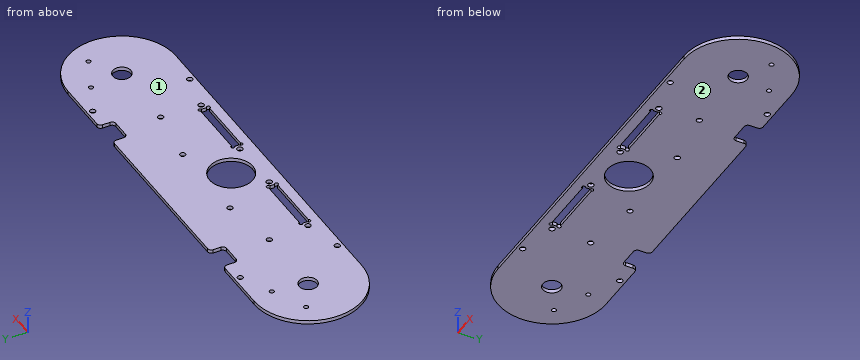
from build123d import *

# Parameters (mm, degrees)
EXTRUDE_1_DEPTH     = 2
SKETCH_2_R          = 1.55
SKETCH_2_R_2        = 12
SKETCH_2_R_3        = 5.025
SKETCH_2_R_4        = 1.25
CUT_EXTRUDE_1_DEPTH = 130.537639318
SKETCH_3_R          = 1.6
SKETCH_3_W          = 34
SKETCH_3_H          = 5
CUT_EXTRUDE_2_DEPTH = 130.537639318
SKETCH_4_W          = 14
SKETCH_4_H          = 8.3
CUT_EXTRUDE_3_DEPTH = 130.537639318
FILLET_1_R          = 2
SKETCH_5_R          = 1
CUT_EXTRUDE_4_DEPTH = 130.537639318


with BuildPart() as part:
    # ｽｹｯﾁ1 → ﾎﾞｽ - 押し出し1 (new body)
    with BuildSketch(Plane.XY):
        with BuildLine():
            Line((-96, -30), (96, -30))
            ThreePointArc((96, -30), (126, 0), (96, 30))
            Line((96, 30), (-96, 30))
            ThreePointArc((-96, 30), (-126, 0), (-96, -30))
        make_face()
    extrude(amount=EXTRUDE_1_DEPTH)

    # ｽｹｯﾁ2 → ｶｯﾄ - 押し出し1 (cut, through all)
    with BuildSketch(Plane.XY.offset(2)):
        with Locations((-56, 0)):
            Circle(SKETCH_2_R)
        with Locations(Location((56, 0, 0), (0, 0, 180))):
            Circle(SKETCH_2_R)
        with Locations((-76, 27)):
            Circle(SKETCH_2_R)
        with Locations((-76, -27)):
            Circle(SKETCH_2_R)
        with Locations(Location((76, 27, 0), (0, 0, 180))):
            Circle(SKETCH_2_R)
        with Locations(Location((76, -27, 0), (0, 0, 180))):
            Circle(SKETCH_2_R)
        with Locations((-24.362267564, 4.80144627)):
            Circle(SKETCH_2_R)
        with Locations(Location((24.362267564, 4.80144627, 0), (0, 0, 180))):
            Circle(SKETCH_2_R)
        with Locations((0, -9)):
            Circle(SKETCH_2_R_2)
        with Locations((-96, 0)):
            Circle(SKETCH_2_R_3)
        with Locations((96, 0)):
            Circle(SKETCH_2_R_3)
        with Locations((-112.152077461, 9.846364808)):
            Circle(SKETCH_2_R_4)
        with Locations((-93.160397784, 18.702330483)):
            Circle(SKETCH_2_R_4)
        with Locations(Location((93.160397784, 18.702330483, 0), (0, 0, 180))):
            Circle(SKETCH_2_R_4)
        with Locations(Location((112.152077461, 9.846364808, 0), (0, 0, 180))):
            Circle(SKETCH_2_R_4)
    extrude(amount=-CUT_EXTRUDE_1_DEPTH, mode=Mode.SUBTRACT)

    # ｽｹｯﾁ3 → ｶｯﾄ - 押し出し2 (cut, through all)
    with BuildSketch(Plane.XY.offset(2)):
        with Locations((55.057299255, -22)):
            Circle(SKETCH_3_R)
        with Locations((15.057299255, -22)):
            Circle(SKETCH_3_R)
        with Locations(Location((-55.057299255, -22, 0), (0, 0, 180))):
            Circle(SKETCH_3_R)
        with Locations(Location((-15.057299255, -22, 0), (0, 0, 180))):
            Circle(SKETCH_3_R)
        with Locations((35.057299255, -22)):
            Rectangle(SKETCH_3_W, SKETCH_3_H)
        with Locations((-35.057299255, -22)):
            Rectangle(SKETCH_3_W, SKETCH_3_H)
    extrude(amount=-CUT_EXTRUDE_2_DEPTH, mode=Mode.SUBTRACT)

    # ｽｹｯﾁ4 → ｶｯﾄ - 押し出し3 (cut, through all)
    with BuildSketch(Plane.XY.offset(2)):
        with Locations((-57.057299255, 25.85)):
            Rectangle(SKETCH_4_W, SKETCH_4_H)
        with Locations((57.057299255, 25.85)):
            Rectangle(SKETCH_4_W, SKETCH_4_H)
    extrude(amount=-CUT_EXTRUDE_3_DEPTH, mode=Mode.SUBTRACT)

    # ﾌｨﾚｯﾄ1
    fillet_1_edges = [part.edges().sort_by_distance(p)[0] for p in [
        (-64.057299255, 21.7, 1),
        (-64.057299255, 30, 1),
        (-50.057299255, 30, 1),
        (-50.057299255, 21.7, 1),
        (50.057299255, 21.7, 1),
        (50.057299255, 30, 1),
        (64.057299255, 30, 1),
        (64.057299255, 21.7, 1),
    ]]
    fillet(fillet_1_edges, radius=FILLET_1_R)

    # ｽｹｯﾁ5 → ｶｯﾄ - 押し出し4 (cut, through all)
    with BuildSketch(Plane.XY.offset(2)):
        with Locations((-51.807299255, -19.75)):
            Circle(SKETCH_5_R)
        with Locations((-51.807299255, -24.25)):
            Circle(SKETCH_5_R)
        with Locations((-18.307299255, -24.25)):
            Circle(SKETCH_5_R)
        with Locations((-18.307299255, -19.75)):
            Circle(SKETCH_5_R)
        with Locations((18.307299255, -19.75)):
            Circle(SKETCH_5_R)
        with Locations((18.307299255, -24.25)):
            Circle(SKETCH_5_R)
        with Locations((51.807299255, -24.25)):
            Circle(SKETCH_5_R)
        with Locations((51.807299255, -19.75)):
            Circle(SKETCH_5_R)
    extrude(amount=-CUT_EXTRUDE_4_DEPTH, mode=Mode.SUBTRACT)


solid = part.part
Can you work these out from the model? Positions are in its coordinate system, mm. Face numbers are marked on the shaded views. Coordinates: 2 decimals unless noted, no trailing zeros. Order: outer loops, then holes, each group sorted by start corner. A loop starts at its lowest first (then second) coordinate and runs counter-clockwise, first axis right, second up. Notation, with made-up numbers: M 71,-20 L 105,-20 A14 cw 105,3 Z; hole C 24,-25.75 d7. An arc over 180 degrees is marked long. Write item = value, one per line.
(1) Suppose I cut it at B-B on x = 41.5. Please give me the cut outline in (y, z), plus the area to 3 significant figures.
Results are:
outline = M -30,0 L -24.5,0 L -24.5,2 L -30,2 Z; M -19.5,0 L 30,0 L 30,2 L -19.5,2 Z
area = 110 mm2
(2) If we mould it in two halves opening along Z, with no side actions, what happens to the marked faces 1 and 2? For each: pulls with the +Z half, pulls with the -Z half, needs draft (parallel to the pull), parting line crosses it, or undercut.
Results are:
face_1 = pulls with the +Z half
face_2 = pulls with the -Z half
(3) I need wall thicknesses on line 1 along Y through (x, z) = (56, 0.15); line 2 along Y through (x, z) = (-76, 1); line 3 along X through (y, z) = (18.5, 1.95). Which ranges of each line are inside material? Lowest first, please. Write a range as [from, to].
Results are:
line_1 = [-30, -23.29], [-20.71, -1.55], [1.55, 21.7]
line_2 = [-30, -28.55], [-25.45, 25.45], [28.55, 30]
line_3 = [-119.62, -94.39], [-91.93, 91.93], [94.39, 119.62]
(4) Suppose I cut it at A-A on x = 0. Please give me the cut outline in (y, z).
Results are:
outline = M -30,0 L -21,0 L -21,2 L -30,2 Z; M 3,0 L 30,0 L 30,2 L 3,2 Z
(5) For pin 1 Ø1.9 at (x, y) = (-55.06, -22) entering from -Z; pin 2 Ø1 at (x, z) = (58.5, 1) entering from +Y; pin 3 Ø5 at (x, y) = (-15.06, -22) entering from -Z, each with a flat end and sliding along its axis, tell me the tip position at first contact or that it passes through.
Results are:
pin_1 = through
pin_2 = 21.7
pin_3 = 0
(6) Suppose I cut it at C-C on z = 1.4. State how many separate pieces and enclosed holes the cut face has, plus the area to 3 significant figures.
Results are:
separate_pieces = 1
enclosed_holes = 21
area = 13,000 mm2
